```python
from build123d import *

# Parameters (mm, degrees)
SKETCH1_W                 = 7.62
SKETCH1_H                 = 7.62
BOSS_EXTRUDE1_DEPTH       = 0.254
SKETCH2_W                 = 7.62
SKETCH2_H                 = 7.62
BOSS_EXTRUDE2_DEPTH       = 15.24
CHAMFER1_SIZE             = 7.62
CHAMFER1_SIZE2            = 4.399409051
CHAMFER2_SIZE             = 3.81
CHAMFER2_SIZE2            = 7.16045777
BOSS_EXTRUDE5_DEPTH       = 12.7
SKETCH7_W                 = 10.16
SKETCH7_H                 = 12.7
BOSS_EXTRUDE7_DEPTH       = 2.54
SWEEP1_START              = 0.02132645
SWEEP1_DEPTH              = 10.16
SWEEP2_START              = -17.80132645
SWEEP2_DEPTH              = 10.16
BOSS_EXTRUDE9_DEPTH       = 0.508
SKETCH12_W                = 11.176
SKETCH12_H                = 5.08
BOSS_EXTRUDE11_DEPTH      = 10.16
BOSS_EXTRUDE12_DEPTH      = 0.508
SKETCH14_W                = 11.176
SKETCH14_H                = 6.35
BOSS_EXTRUDE13_DEPTH      = 10.16
SKETCH17_W                = 30.48
SKETCH17_H                = 15.24
BOSS_EXTRUDE16_DEPTH      = 40.64
CHAMFER10_SIZE            = 15.08
CHAMFER10_SIZE2           = 4.899789019
CHAMFER11_SIZE            = 4.92
CHAMFER11_SIZE_2          = 18.361689973
CHAMFER12_SIZE            = 2.38
CHAMFER12_SIZE2           = 2.886919979
CUT_EXTRUDE1_DEPTH        = 12.7
BOSS_EXTRUDE17_DEPTH      = 12.7
BOSS_EXTRUDE17_DEPTH_BACK = 5.08
CHAMFER14_SIZE            = 10.16
CHAMFER14_SIZE_2          = 37.917636205
BOSS_EXTRUDE18_DEPTH      = 12.7
SKETCH22_W                = 30.48
SKETCH22_H                = 5.030470453
BOSS_EXTRUDE19_DEPTH      = 0.127


# Read off the part's stored shape, not the designer's step: Sweep1, Sweep2
with BuildPart() as part:
    # Sketch1 → Boss-Extrude1 (new body)
    with BuildSketch(Plane(origin=(0, 0, 0), x_dir=(1, 0, 0), z_dir=(0, 1, 0))):
        with Locations((3.81, 3.81)):
            Rectangle(SKETCH1_W, SKETCH1_H)
    extrude(amount=BOSS_EXTRUDE1_DEPTH)

    # Sketch2 → Boss-Extrude2 (add)
    with BuildSketch(Plane.XZ):
        Polygon((7.62, -7.62), (3.81, -7.62), (3.81, -19.05), (13.97, -19.05), (13.97, 11.43), (3.81, 11.43), (3.81, 0), (7.62, 0), align=None)
        Polygon((3.81, -19.05), (3.81, -7.62), (0, -7.62), (0, 0), (3.81, 0), (3.81, 11.43), (-11.525577389, 11.43), (-11.525577389, -19.05), align=None)
        with Locations((3.81, -3.81)):
            Rectangle(SKETCH2_W, SKETCH2_H)
    extrude(amount=BOSS_EXTRUDE2_DEPTH)

    # Chamfer1
    chamfer1_edges = [part.edges().sort_by_distance(p)[0] for p in [
        (-11.525577389, 0, -3.81),
    ]]
    chamfer1_side = [part.faces().sort_by_distance(p)[0] for p in [
        (1.222211305, 0, -18.652626767),
    ]]
    chamfer(chamfer1_edges, length=CHAMFER1_SIZE, length2=CHAMFER1_SIZE2, reference=chamfer1_side[0])

    # Chamfer2
    chamfer2_edges = [part.edges().sort_by_distance(p)[0] for p in [
        (-11.525577389, -4.399409051, -3.81),
    ]]
    chamfer2_side = [part.faces().sort_by_distance(p)[0] for p in [
        (-7.715577389, -2.199704526, -3.81),
    ]]
    chamfer(chamfer2_edges, length=CHAMFER2_SIZE, length2=CHAMFER2_SIZE2, reference=chamfer2_side[0])

    # Sketch3 → Boss-Extrude5 (add)
    with BuildSketch(Plane.XZ.offset(15.24)):
        Polygon((1.222211305, -13.998435267), (10.045655072, -8.904217634), (10.045655072, 1.284217634), (1.222211305, 6.378435267), (-7.601232461, 1.284217634), (-7.601232461, -8.904217634), align=None)
    extrude(amount=BOSS_EXTRUDE5_DEPTH)

    # Sketch7 → Boss-Extrude7 (add)
    with BuildSketch(Plane(origin=(13.97, 0, 0), x_dir=(0, 0, -1), z_dir=(1, 0, 0))):
        Polygon((-3.81, -7.62), (-0.02132645, -7.62), (-0.02132645, -2.54), (-10.18132645, -2.54), (-10.18132645, -7.62), align=None)
        Polygon((-3.83132645, -15.24), (-3.81, -7.62), (-10.18132645, -7.62), (-10.18132645, -15.24), align=None)
        Polygon((-0.02132645, -15.24), (-0.02132645, -7.62), (-3.81, -7.62), (-3.83132645, -15.24), align=None)
        with Locations((12.72132645, -8.89)):
            Rectangle(SKETCH7_W, SKETCH7_H)
    extrude(amount=BOSS_EXTRUDE7_DEPTH)

    # Sweep1 outline → Sweep1 (add)
    with BuildSketch(Plane.XY.offset(SWEEP1_START)):
        Polygon((16.51, -15.24), (29.045138309, -27.775138309), (29.045138309, -15.075138309), (16.51, -2.54), align=None)
    extrude(amount=SWEEP1_DEPTH)

    # Sweep2 outline → Sweep2 (add)
    with BuildSketch(Plane.XY.offset(SWEEP2_START)):
        Polygon((16.51, -2.54), (16.51, -15.24), (29.030018127, -27.760018127), (29.030018127, -15.060018127), align=None)
    extrude(amount=SWEEP2_DEPTH)

    # Chamfer5
    # the kernel refuses this chamfer: 14.368409794, 10.16 mm, written as the material it takes off along each edge
    with BuildSketch(Plane(origin=(29.045138309, -27.775138309, 0.02132645), x_dir=(-0.7459142715976749, 0.6660419652145878, 0), z_dir=(0, 0, 1)), Plane(origin=(29.030018127, -27.760018127, -17.80132645), x_dir=(-0.7459142715976752, 0.6660419652145875, 0), z_dir=(0, 0, 1))) as chamfer5_piece_1:
        with BuildLine():
            Line((10.176243016, 0), (9.537503791, -11.29142094))
            Line((9.537503791, -11.29142094), (9.323151752, -11.482820218))
            ThreePointArc((9.323151752, -11.482820218), (4.705969637, -5.701770021), (-0.214352039, -0.191399278))
            Line((-0.214352039, -0.191399278), (0.016230053, 0.286909507))
            ThreePointArc((0.016230053, 0.286909507), (5.088121508, 0), (10.192473069, 0.286909507))
            Line((10.192473069, 0.286909507), (10.176243016, 0))
        make_face()
    extrude(amount=10.16, mode=Mode.SUBTRACT)

    # Sketch10 → Boss-Extrude9 (add)
    with BuildSketch(Plane(origin=(6.985, 6.985, 0), x_dir=(0, 0, -1), z_dir=(0.7071067811865389, 0.7071067811865561, 0))):
        Polygon((12.72132645, -21.73350196), (18.30932645, -21.73350196), (18.30932645, -26.81350196), (7.13332645, -26.81350196), (7.13332645, -21.73350196), align=None)
    extrude(amount=BOSS_EXTRUDE9_DEPTH)

    # Sketch12 → Boss-Extrude11 (add)
    with BuildSketch(Plane(origin=(7.344210245, 7.344210245, 0), x_dir=(0, 0, -1), z_dir=(0.707106781186539, 0.707106781186556, 0))):
        with Locations((12.72132645, -24.27350196)):
            Rectangle(SKETCH12_W, SKETCH12_H)
    extrude(amount=-BOSS_EXTRUDE11_DEPTH)

    # Sketch13 → Boss-Extrude12 (add)
    with BuildSketch(Plane(origin=(6.985, 6.985, 0), x_dir=(0, 0, -1), z_dir=(0.7071067811865389, 0.7071067811865562, 0))):
        Polygon((-5.10132645, -21.744193544), (-10.68932645, -21.744193544), (-10.68932645, -28.094193544), (0.48667355, -28.094193544), (0.48667355, -21.744193544), align=None)
    extrude(amount=BOSS_EXTRUDE12_DEPTH)

    # Sketch14 → Boss-Extrude13 (add)
    with BuildSketch(Plane(origin=(7.344210245, 7.344210245, 0), x_dir=(0, 0, -1), z_dir=(0.7071067811865388, 0.7071067811865562, 0))):
        with Locations((-5.10132645, -24.919193544)):
            Rectangle(SKETCH14_W, SKETCH14_H)
    extrude(amount=-BOSS_EXTRUDE13_DEPTH)

    # Sketch17 → Boss-Extrude16 (add)
    with BuildSketch(Plane(origin=(13.97, 0, 0), x_dir=(0, 0, -1), z_dir=(1, 0, 0))):
        with Locations((3.81, -7.62)):
            Rectangle(SKETCH17_W, SKETCH17_H)
    extrude(amount=-BOSS_EXTRUDE16_DEPTH)

    # Chamfer10
    chamfer10_edges = [part.edges().sort_by_distance(p)[0] for p in [
        (-26.67, 0, -3.81),
    ]]
    chamfer10_side = [part.faces().sort_by_distance(p)[0] for p in [
        (-26.67, -7.62, -3.81),
    ]]
    chamfer(chamfer10_edges, length=CHAMFER10_SIZE, length2=CHAMFER10_SIZE2, reference=chamfer10_side[0])

    # Chamfer11
    # the kernel refuses this chamfer: 18.361689973, 4.92 mm, written as the material it takes off along each edge
    with BuildSketch(Plane(origin=(-26.67, -15.24, -66.730196419), x_dir=(-0.13751244702129126, 0.990500038825954, 0), z_dir=(0, 0, 1))) as chamfer11_piece_1:
        Polygon((CHAMFER11_SIZE * 0.990500038826, -CHAMFER11_SIZE * 0.137512447021), (-CHAMFER11_SIZE_2 * 0.137512447023, -CHAMFER11_SIZE_2 * 0.990500038839), (0, 0), align=None)
    extrude(amount=125.840392838, mode=Mode.SUBTRACT)

    # Chamfer12
    chamfer12_edges = [part.edges().sort_by_distance(p)[0] for p in [
        (-21.770210981, 0, -3.81),
    ]]
    chamfer12_side = [part.faces().sort_by_distance(p)[0] for p in [
        (-4.334202117, 0, -3.81),
    ]]
    chamfer(chamfer12_edges, length=CHAMFER12_SIZE, length2=CHAMFER12_SIZE2, reference=chamfer12_side[0])

    # Sketch19 → Cut-Extrude1 (cut)
    with BuildSketch(Plane.XZ.offset(27.94)):
        Polygon((-7.601232461, 1.284217634), (-7.601232461, -8.904217634), (1.222211305, -13.998435267), (10.045655072, -8.904217634), (10.045655072, 1.284217634), (1.222211305, 6.378435267), align=None)
    extrude(amount=-CUT_EXTRUDE1_DEPTH, mode=Mode.SUBTRACT)

    # Sketch20 → Boss-Extrude17 (add, two sides: drawn at the far end of the back side and taken through both)
    with BuildSketch(Plane(origin=(0, -15.24, 0), x_dir=(-1, 0, 0), z_dir=(0, -1, 0)).offset(-BOSS_EXTRUDE17_DEPTH_BACK)):
        Polygon((8.308310027, -8.89), (19.306832655, -2.54), (19.306832655, 10.16), (8.308310027, 16.51), (-2.690212601, 10.16), (-2.690212601, -2.54), align=None)
    extrude(amount=BOSS_EXTRUDE17_DEPTH + BOSS_EXTRUDE17_DEPTH_BACK)

    # Chamfer14
    # the kernel refuses this chamfer: 37.917636205, 10.16 mm, written as the material it takes off along each edge
    with BuildSketch(Plane(origin=(-19.306832655, -27.94, 101.001543824), x_dir=(-0.13751244702129076, 0.9905000388259542, 0), z_dir=(0, 0, -1))) as chamfer14_piece_1:
        Polygon((CHAMFER14_SIZE * 0.990500038826, CHAMFER14_SIZE * 0.137512447021), (-CHAMFER14_SIZE_2 * 0.137512447021, CHAMFER14_SIZE_2 * 0.990500038823), (0, 0), align=None)
    extrude(amount=209.623087649, mode=Mode.SUBTRACT)

    # Sketch21 → Boss-Extrude18 (add)
    with BuildSketch(Plane(origin=(0, -15.24, 0), x_dir=(-1, 0, 0), z_dir=(0, -1, 0))):
        Polygon((8.308310027, -5.08), (16.007275866, -0.635), (16.007275866, 8.255), (8.308310027, 12.7), (0.609344187, 8.255), (0.609344187, -0.635), align=None)
    extrude(amount=BOSS_EXTRUDE18_DEPTH)

    # Sketch22 → Boss-Extrude19 (add)
    with BuildSketch(Plane(origin=(-19.691340818, 6.398104477, 0), x_dir=(0, 0, 1), z_dir=(-0.9510565162951544, 0.30901699437494484, 0))):
        with Locations((-3.81, -12.129520369)):
            Rectangle(SKETCH22_W, SKETCH22_H)
    extrude(amount=BOSS_EXTRUDE19_DEPTH)


solid = part.part
```
Here's how the part is built. I have some questions about the finished solid (model axes, mm). A direction names the side the tool comes from. Give positions to 0.01 mm unless a question says otherwise; leave off trailing zeros. Order: outer loops, then holes, each group sorted by start corner. A loop starts at its lowest first (then second) coordinate and runs counter-clockwise, first axis right, second up. Notation, with made-up numbers: (52, -4.75) - (110, -4.75) arc R24 ccw to (110, 24.25) - close; hole circle Ø2 at (62.5, 7). An arc over 180 degrees is marked (long way). Answer as a JSON object with one key per item and string values. Group by question number.
Item 1: Please list where these lines run through material, in increasing order: probe 1 along Y at (x, z) = (-5.5, 8.5); probe 2 along X at (y, z) = (-22, -7.5); probe 3 along Y at (x, z) = (-1.5, -4).
Item 2: If we mould it in two halves opening along X, with no side actions, what happens to faces 6 (the flat face through (-4, -9, -19.05)), 7 (the flat face through (-4.405, -25.084, 2.826)), 8 (the flat face through (24.976, -17.445, -12.792)), 9 (the flat face through (17, -9, 0.021))? For each: pulls with the +X half, pulls with the -X half, needs draft (parallel to the pull), parting line crosses it, or undercut.
Item 3: If we section it at A-A on x = 24.5: Please give me the cut outline in (y, z), and give its area (3 significant figures).
Item 4: If we section it at C-C on y = -5.5: Please give me the cut outline in (x, z).
Item 5: For P1, Ø6.5, axis at x = 19.5, y = -7.5, coming from the +Z side; P2, Ø1.3, axis at x = 14.5, z = -15, coming from the +Y side; P3, Ø3.5, axis at x = 24, y = -11, coming from the -Z side; P4, Ø1.5, axis at x = 6, y = -17, coming from the +Z side, each with a flat end and sliding along its axis, tell me the tip position at first contact or that it passes through.
Item 6: Which directions (+Z, -Z, +X, -X, +Y, -Y) give clear straight access to the entire face, cutting with the end or side of a thin tool? Please do faces 1 (the flat face through (24, -16, -7.641)), 2 (the flat face through (-2.89, -18.46, -13.38)), 3 (the flat face through (-20.66, -11.93, -4.02)), 4 (the flat face through (-2.73, -18.46, 5.67)), 5 (the flat face through (-13.248, -19.403, -10.336)).
Item 7: If we section it at B-B on z = -3: Please give me the cut outline in (x, y).
Item 8: If we section it at D-D on x = 2: Please give me the cut outline in (y, z), and give its area (3 significant figures).
Result set:
{
 "1": {"probe 1": "-15.24 to 0", "probe 2": "-16.01 to 2.69", "probe 3": "-27.94 to 0"},
 "2": {"face 6": "needs draft", "face 7": "undercut", "face 8": "pulls with the +X half", "face 9": "undercut"},
 "3": {"outline": "(-17.95, 0.02) - (-15.23, 0.02) - (-15.23, -0.49) - (-9.81, -0.49) - (-9.81, 10.69) - (-15.23, 10.69) - (-15.23, 10.18) - (-17.95, 10.18) - close; (-17.92, -17.8) - (-13.42, -17.8) - (-13.42, -18.31) - (-9.81, -18.31) - (-9.81, -7.13) - (-13.42, -7.13) - (-13.42, -7.64) - (-17.92, -7.64) - close", "area": "174 mm²"},
 "4": {"outline": "(-23.69, -19.05) - (13.97, -19.05) - (13.97, -17.8) - (19.47, -17.8) - (19.47, -7.64) - (13.97, -7.64) - (13.97, 0.02) - (19.47, 0.02) - (19.47, 10.18) - (13.97, 10.18) - (13.97, 11.43) - (-23.69, 11.43) - close"},
 "5": {"P1": "z = 10.69", "P2": "y = 0", "P3": "z = -18.31", "P4": "through"},
 "6": {"face 1": "+X, -Y", "face 2": "-Z, -Y", "face 3": "-X, -Y", "face 4": "+Z, -Y", "face 5": "-Y"},
 "7": {"outline": "(-25.25, -10.7) - (-19.31, -12.29) - (-19.31, -17.78) - (-16.01, -18.66) - (-16.01, -27.94) - (-0.61, -27.94) - (-0.61, -22.79) - (2.69, -23.67) - (2.69, -15.24) - (13.97, -15.24) - (13.97, 0) - (7.62, 0) - (7.62, 0.25) - (0, 0.25) - (0, 0) - (-19.39, 0) - (-22.66, -2.75) - (-22.78, -2.71) - (-24.34, -7.49) - (-24.22, -7.53) - close"},
 "8": {"outline": "(-23.49, -10.56) - (-15.24, -10.56) - (-15.24, -19.05) - (0, -19.05) - (0, -7.62) - (0.25, -7.62) - (0.25, 0) - (0, 0) - (0, 11.43) - (-15.24, 11.43) - (-15.24, 2.94) - (-23.49, 2.94) - close", "area": "578 mm²"}
}
